from build123d import *

# Parameters (mm, degrees)
SKETCH_1_R          = 3.25
EXTRUDE_1_DEPTH     = 6
SKETCH_2_R          = 6
CUT_EXTRUDE_1_DEPTH = 2


with BuildPart() as part:
    # Эскиз1 → Бобышка-Вытянуть1 (new body)
    with BuildSketch(Plane(origin=(0, 0, 0), x_dir=(1, 0, 0), z_dir=(0, 1, 0))):
        with BuildLine():
            Line((-4.939643838, -18.225455779), (-8.542011418, -41.199499519))
            Line((-8.542011418, -41.199499519), (-10, -41.199499519))
            Line((-10, -41.199499519), (-10, 0))
            ThreePointArc((-10, 0), (0, 10), (10, 0))
            Line((10, 0), (10, -41.199499519))
            Line((10, -41.199499519), (8.542011418, -41.199499519))
            Line((8.542011418, -41.199499519), (4.939643838, -18.225455779))
            ThreePointArc((4.939643838, -18.225455779), (0, -14), (-4.939643838, -18.225455779))
        make_face()
        Circle(SKETCH_1_R, mode=Mode.SUBTRACT)
    extrude(amount=EXTRUDE_1_DEPTH)

    # Эскиз2 → Вырез-Вытянуть1 (cut)
    with BuildSketch(Plane.XZ):
        Circle(SKETCH_2_R)
    extrude(amount=-CUT_EXTRUDE_1_DEPTH, mode=Mode.SUBTRACT)


solid = part.part
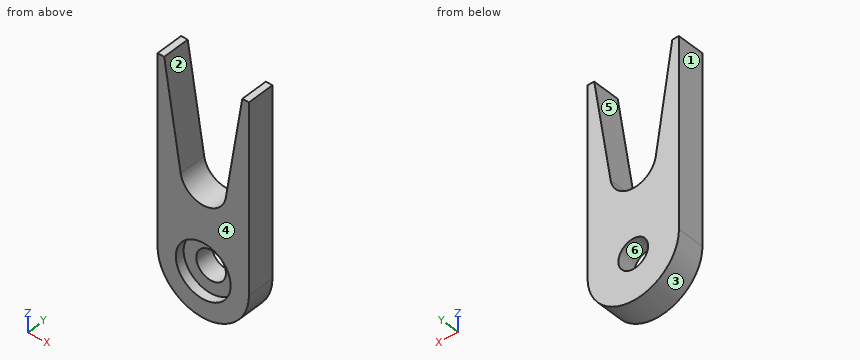
Could you check a few things on this model? Use its own coordinates, in mm. Face numbers are marked on the shaded views. A direction names the side the tool comes from. Give positions to 0.01 mm unless a question says otherwise; leave off trailing zeros. Order: outer loops, then holes, each group sorted by start corner. A loop starts at its lowest first (then second) coordinate and runs counter-clockwise, first axis right, second up.
1. For the marked faces 1 and 2, which set-ups out of +Z, -Z, +X, -X, +Y, -Y let a thin tool reach every point of the face, with its end or its side?
2. We'd pull the mould along X, two halves only. Please class the marked faces 3, 4, 5 and 6: pulls with the +X half, pulls with the -X half, needs draft (parallel to the pull), parting line crosses it, or undercut.
3. Will these pins go through, and if not, where does the flat tip stop? P1, Ø4, axis at x = 0, z = 0, coming from the +Y side; P2, Ø2, axis at x = 2, y = 5, coming from the -Z side; P3, Ø1.5, axis at x = -2.5, z = 0.5, coming from the -Y side.
4. Suppose I cut it at B-B (y = 4.8). List the corners of the cut face in (x, z) for me.
5. Suppose I cut it at D-D (z = -1). List the corners of the cut face in (x, y) for me, plus the area to 3 significant figures.
6. Suppose I cut it at C-C (z = 19.5). List the corners of the cut face in (x, y) for me.
7. I need wall thicknesses on L1, parallel to X at y = 4.4, z = 0; L2, parallel to Z at x = 0, y = 3.75; L3, parallel to Z at x = 0, y = 0.55. Which ranges of each line are inside material? Lowest first, please.
8. Suppose I cut it at A-A (x = 0). List the corners of the cut face in (y, z) for me, plus the area to 3 significant figures.
Solved:
1. face 1: +Z, -Z, -X, +Y, -Y
1. face 2: +Z, +Y, -Y
2. face 3: parting line crosses it
2. face 4: needs draft
2. face 5: undercut
2. face 6: undercut
3. P1: passes through
3. P2: stops at z = -9.95
3. P3: stops at y = 2
4. outline: (-10, 0) arc R10 ccw to (10, 0) - (10, 41.2) - (8.54, 41.2) - (4.94, 18.23) arc R5 cw to (-4.94, 18.23) - (-8.54, 41.2) - (-10, 41.2) - close; hole circle Ø6.5 at (0, 0)
5. outline: (-9.95, 0) - (-5.92, 0) - (-5.92, 2) - (-3.09, 2) - (-3.09, 6) - (-9.95, 6) - close; (3.09, 2) - (5.92, 2) - (5.92, 0) - (9.95, 0) - (9.95, 6) - (3.09, 6) - close
5. area: 71.0 mm2
6. outline: (-10, 0) - (-5.14, 0) - (-5.14, 6) - (-10, 6) - close; (5.14, 0) - (10, 0) - (10, 6) - (5.14, 6) - close
7. L1: x = -10 to -3.25, 3.25 to 10
7. L2: z = -10 to -3.25, 3.25 to 14
7. L3: z = -10 to -6, 6 to 14
8. outline: (0, -10) - (6, -10) - (6, -3.25) - (2, -3.25) - (2, -6) - (0, -6) - close; (0, 6) - (2, 6) - (2, 3.25) - (6, 3.25) - (6, 14) - (0, 14) - close
8. area: 94.0 mm2
